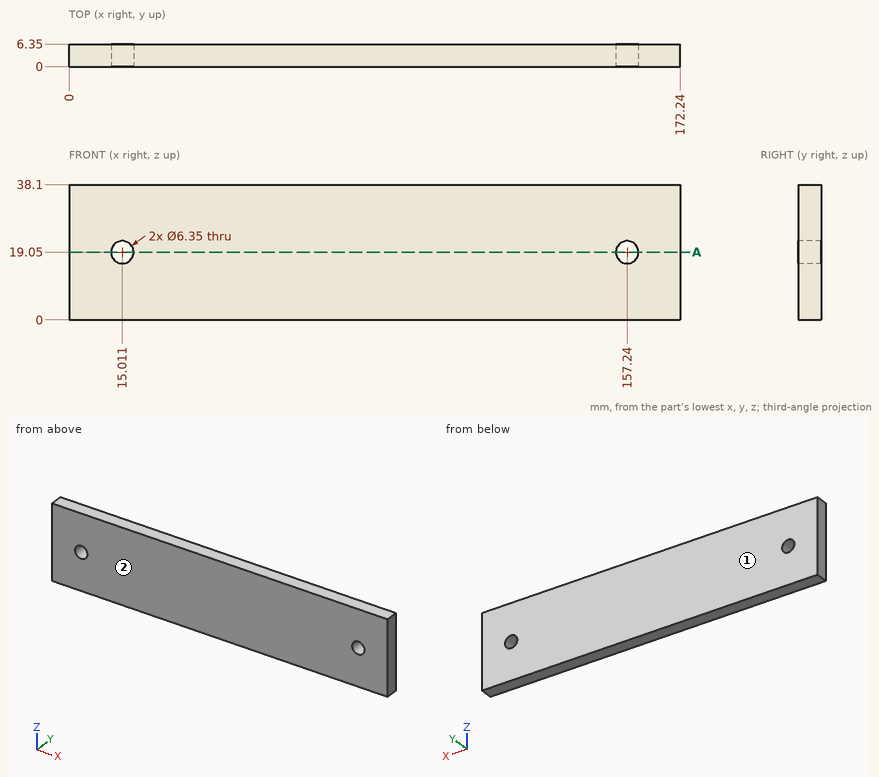
Geometry: see drawing. Coordinates: mm, zero at the bounding-box minimum. Coordinates: 2 decimals unless noted, no trailing zeros. Put each result on its own line as item: value. Start each with the question number.
1) Cut plane A-A on z = 19.05. Give the number of separate pieces and of enclosed holes in the cut face, then the cut area to 3 significant figures.
2) Ray query, L1, parallel to X at y = 4.5, z = 19.05 (1 decimal). Return the intervals inside material, ascending. Write a range as from..to.
3) Pull-direction query (Y, two-part tool) for the marked faces 1 and 2; classes: pulls with the +Y half, pulls with the -Y half, needs draft (parallel to the pull), parting line crosses it, or undercut.
The answers:
1. separate pieces: 3
1. enclosed holes: 0
1. area: 1,010 mm²
2. L1: x = 0..11.8, 18.2..154.1, 160.4..172.2
3. face 1: pulls with the +Y half
3. face 2: pulls with the -Y half
